Autodesk Inventor part; units mm, degrees
ref_plane "YZ Plane" through (0, 0, 0) normal (1, 0, 0) x (0, 1, 0)
ref_plane "XZ Plane" through (0, 0, 0) normal (0, 1, 0) x (-1, 0, 0)
ref_plane "XY Plane" through (0, 0, 0) normal (0, 0, 1) x (1, 0, 0)
sketch "Sketch1" plane through (0, 0, 0) normal (1, 0, 0) x (0, 1, 0)
  circle A0 centre (0, 0) radius 4
  dimension "d0" = 8
extrude "Extrusion1" add sketch "Sketch1" along normal mid plane 13.8
sketch "Sketch2" plane through (6.9, 0, 0) normal (1, 0, 0) x (0, 0, -1)
  circle A0 centre (0, 0) radius 3
  dimension "d3" = 6
extrude "Extrusion2" add sketch "Sketch2" along normal blind 0.4
sketch "Sketch3" plane through (7.3, 0, 0) normal (1, 0, 0) x (0, 0, -1)
  circle A0 centre (0, 0) radius 0.5
  dimension "d6" = 1
extrude "Extrusion3" add sketch "Sketch3" along normal blind 4
properties part number "AM0820 Stepper"
The model under review builds one solid part; all positions refer to its coordinate system, in mm. A direction names the side the tool comes from. Give positions to 0.01 mm unless a question says otherwise; leave off trailing zeros. Write each loop counter-clockwise with the first axis right and the second up, starting at its lowest first coordinate (ties: lowest second). Pieces come first, ordered by that corner, then holes. Notation, with made-up numbers: (38, 45.5) -> (72, 45.5) arc R17 cw to (72, 68.5) -> close; hole circle Ø5 at (4.25, -10.5). An arc over 180 degrees is marked (long way). Answer in a Markdown table with one row per item.
1) Add section A-A on z = 0. State the section outline as (x, y) points, plus the area to 3 significant figures.
Worked answers:
| item | result |
|---|---|
| outline | (-6.9, -4) -> (6.9, -4) -> (6.9, -3) -> (7.3, -3) -> (7.3, -0.5) -> (11.3, -0.5) -> (11.3, 0.5) -> (7.3, 0.5) -> (7.3, 3) -> (6.9, 3) -> (6.9, 4) -> (-6.9, 4) -> close |
| area | 117 mm² |
2) For L1, parallel to X at y = -2.25, z = 2.5; L2, parallel to X at y = -0.5, z = 2.75; L3, parallel to Y at x = 3, z = -2.25, list the stretches that pass through material, from the lowest coordinate up. Write a range as [from, to].
Worked answers:
| item | result |
|---|---|
| L1 | [-6.9, 6.9] |
| L2 | [-6.9, 7.3] |
| L3 | [-3.31, 3.31] |
3) Add section D-D on z = -2. State the section outline as (x, y) points, plus the area to 3 significant figures.
Worked answers:
| item | result |
|---|---|
| outline | (-6.9, -3.46) -> (6.9, -3.46) -> (6.9, -2.24) -> (7.3, -2.24) -> (7.3, 2.24) -> (6.9, 2.24) -> (6.9, 3.46) -> (-6.9, 3.46) -> close |
| area | 97.4 mm² |
4) Add section C-C on x = 4. State the section outline as (y, z) points, plus the area to 3 significant figures.
Worked answers:
| item | result |
|---|---|
| outline | circle Ø8 at (0, 0) |
| area | 50.3 mm² |
5) Clearance check with flat-ended pins moving along their axes: P1, Ø1, axis at x = 7, y = -3, coming from the +Z side; P2, Ø2, axis at y = -1.5, z = 1.5, coming from the +X side; P3, Ø3, axis at x = 7.5, y = -2.5, coming from the -Z side. State where each tip first meets the part, or that it passes through.
Worked answers:
| item | result |
|---|---|
| P1 | z = 3.11 |
| P2 | x = 7.3 |
| P3 | z = -3.84 |
6) Tool access review of faces 1 (the cylindrical face through (9.272, 0.488, 0.108)), 2 (the flat face through (11.3, 0, 0)): name each direction out of +Z, -Z, +X, -X, +Y, -Y from which nothing blocks a thin tool from reaching the whole face with its end or side.
Worked answers:
| item | result |
|---|---|
| face 1 | +X |
| face 2 | +Z, -Z, +X, +Y, -Y |
